Input: part model. Units: mm. Frame: model coordinates. A direction names the side the tool comes from. Coordinates: 2 decimals unless noted, no trailing zeros. Order: outer loops, then holes, each group sorted by start corner. A loop starts at its lowest first (then second) coordinate and runs counter-clockwise, first axis right, second up. Notation, with made-up numbers: M 47.5,64.5 L 63.5,64.5 A10 ccw 63.5,68.5 Z; hole C 40.5,72.25 d2. An arc over 180 degrees is marked long. Answer in a Markdown table with one row per item.
from build123d import *

# Parameters (mm, degrees)
F0_W     = 203.2
F0_H     = 203.2
F0_W_2   = 196.85
F0_H_2   = 196.85
F1_DEPTH = 50.8
F2_DEPTH = 3.175
F3_W     = 203.2
F3_H     = 1.5875
F5_DEPTH = 3.175
F4_W     = 203.2
F4_H     = 1.5875
F6_DEPTH = 3.175


with BuildPart() as f1:
    # F0 (on Top) → F1 (new body)
    with BuildSketch(Plane.XY):
        Rectangle(F0_W, F0_H)
        Rectangle(F0_W_2, F0_H_2, mode=Mode.SUBTRACT)
    extrude(amount=F1_DEPTH)

    # F0 (on Top) → F2 (join)
    with BuildSketch(Plane.XY):
        Rectangle(F0_W_2, F0_H_2)
    extrude(amount=F2_DEPTH)

    # F3 (on face) → F5 (join)
    with BuildSketch(Plane(origin=(-101.6, 0, 0), x_dir=(0, -1, 0), z_dir=(-1, 0, 0))):
        with Locations((0, 34.660417)):
            Rectangle(F3_W, F3_H)
        with Locations((0, 33.072917)):
            Rectangle(F3_W, F3_H)
        with Locations((0, 17.727083)):
            Rectangle(F3_W, F3_H)
        with Locations((0, 16.139583)):
            Rectangle(F3_W, F3_H)
    extrude(amount=F5_DEPTH)

    # F4 (on face) → F6 (join)
    with BuildSketch(Plane.YZ.offset(101.6)):
        with Locations((0, 34.660417)):
            Rectangle(F4_W, F4_H)
        with Locations((0, 33.072917)):
            Rectangle(F4_W, F4_H)
        with Locations((0, 17.727083)):
            Rectangle(F4_W, F4_H)
        with Locations((0, 16.139583)):
            Rectangle(F4_W, F4_H)
    extrude(amount=F6_DEPTH)


solid = f1.part
1) Contact query for flat-ended pins moving along their axis: pin 1 (2 mm diameter, centred on x = 32.5, y = -21.5, fed in from +Z) (3 decimals); pin 2 (1.6 mm diameter, centred on x = 102.5, y = -10.5, fed in from -Z); pin 3 (1 mm diameter, centred on x = -103, y = 5.5, fed in from +Z); pin 4 (17 mm diameter, centred on y = 37, z = 42.5, fed in from +X) (3 decimals). Output: stop coordinate, or through.
Resolved:
| item | result |
|---|---|
| pin 1 | stops at z = 3.175 |
| pin 2 | stops at z = 15.35 |
| pin 3 | stops at z = 35.45 |
| pin 4 | stops at x = 104.775 |
2) Cut plane C-C, the plane y = 63. Output: boundary loops of the cut face in (x, z) (3 decimals).
Resolved:
| item | result |
|---|---|
| outline | M -104.775,15.346 L -101.6,15.346 L -101.6,0 L 101.6,0 L 101.6,15.346 L 104.775,15.346 L 104.775,18.521 L 101.6,18.521 L 101.6,32.279 L 104.775,32.279 L 104.775,35.454 L 101.6,35.454 L 101.6,50.8 L 98.425,50.8 L 98.425,3.175 L -98.425,3.175 L -98.425,50.8 L -101.6,50.8 L -101.6,35.454 L -104.775,35.454 L -104.775,32.279 L -101.6,32.279 L -101.6,18.521 L -104.775,18.521 Z |
3) Cut plane A-A, the plane x = 92.5. Output: boundary loops of the cut face in (y, z) (3 decimals), and give its area (3 significant figures).
Resolved:
| item | result |
|---|---|
| outline | M -101.6,0 L 101.6,0 L 101.6,50.8 L 98.425,50.8 L 98.425,3.175 L -98.425,3.175 L -98.425,50.8 L -101.6,50.8 Z |
| area | 948 mm2 |
4) Cut plane B-B, the plane z = 9.5. Output: boundary loops of the cut face in (x, y) (3 decimals).
Resolved:
| item | result |
|---|---|
| outline | M -101.6,-101.6 L 101.6,-101.6 L 101.6,101.6 L -101.6,101.6 Z; hole M -98.425,-98.425 L 98.425,-98.425 L 98.425,98.425 L -98.425,98.425 Z |
5) Reachability of faces 4 (the face through (101.6, -1, 43)), 5 (the face through (101.6, -1, 25)), 6 (the face through (-101.6, -1, 43)), 7 (the face through (101.6, -1, 8)), 8 (the face through (98.425, -1, 27)) from +Z, -Z, +X, -X, +Y, -Y: full face, straight path, thin tool, end or side. Return the list, or none.
Resolved:
| item | result |
|---|---|
| face 4 | +Z, +X, +Y, -Y |
| face 5 | +X, +Y, -Y |
| face 6 | +Z, -X, +Y, -Y |
| face 7 | -Z, +X, +Y, -Y |
| face 8 | +Z |
6) Mould query, pull axis Y, two halves, no side actions, for faces 1 (the face through (-1, 101.6, 25)), 2 (the face through (-1, 1, 3.175)), 3 (the face through (-101.6, -1, 25)). Classes: +Y half, -Y half, draft (parallel to the pull), parting line (faces both ways), or undercut.
Resolved:
| item | result |
|---|---|
| face 1 | +Y half |
| face 2 | undercut |
| face 3 | draft |
7) Material intervals for probe 1 along Y at (x, z) = (-24, 36.5) (3 decimals); probe 2 along Z at (x, y) = (-62.5, 22) (3 decimals), sorted ascending.
Resolved:
| item | result |
|---|---|
| probe 1 | y = -101.6 to -98.425, 98.425 to 101.6 |
| probe 2 | z = 0 to 3.175 |
